Here's the drawing with two shaded views (mm, measured from the low corner). I have some questions. Give positions to 0.01 mm unless a question says otherwise; leave off trailing zeros. Loops run counter-clockwise (first coordinate to the right, second up) from the corner with the lowest first, then second, coordinate; pieces in that order, holes last. Notation, with made-up numbers: M -32.5,79.5 L 11.5,79.5 A25 ccw 11.5,97.5 Z; hole C 37,53 d4. An arc over 180 degrees is marked long. Write item = value, one per line. Start each with the question number.
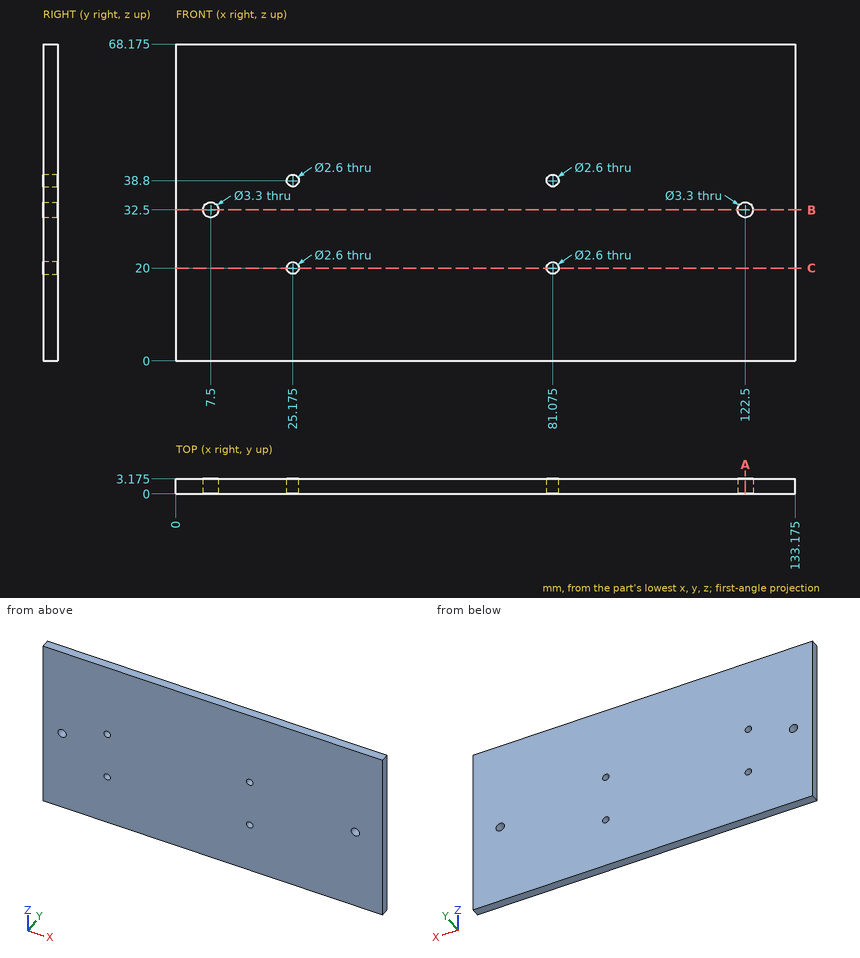
Q1. If we section it at B-B, the plane z = 32.5: List the corners of the cut face in (x, y) for me (3 decimals), then the cut area to 3 significant figures.
Q2. If I drill on line 1 along X through (y, z) = (1.15, 32.5) (3 decimals); line 2 along X through (y, z) = (1.15, 38.8) (3 decimals), over which ranges is the centre line in solid material (lowest first)?
Q3. If we section it at C-C, the plane z = 20: List the corners of the cut face in (x, y) for me (3 decimals).
Q4. Will this pin go through, and if not, where does the flat tip stop? pin 1 (1.6 mm diameter, centred on x = 25.175, z = 38.8, fed in from -Y).
Q5. If we section it at A-A, the plane x = 122.5: List the corners of the cut face in (y, z) for me (3 decimals).
Resolved:
q1.outline = M 0,0 L 5.85,0 L 5.85,3.175 L 0,3.175 Z; M 9.15,0 L 120.85,0 L 120.85,3.175 L 9.15,3.175 Z; M 124.15,0 L 133.175,0 L 133.175,3.175 L 124.15,3.175 Z
q1.area = 402 mm²
q2.line_1 = 0 to 5.85, 9.15 to 120.85, 124.15 to 133.175
q2.line_2 = 0 to 23.875, 26.475 to 79.775, 82.375 to 133.175
q3.outline = M 0,0 L 23.875,0 L 23.875,3.175 L 0,3.175 Z; M 26.475,0 L 79.775,0 L 79.775,3.175 L 26.475,3.175 Z; M 82.375,0 L 133.175,0 L 133.175,3.175 L 82.375,3.175 Z
q4.pin_1 = through
q5.outline = M 0,0 L 3.175,0 L 3.175,30.85 L 0,30.85 Z; M 0,34.15 L 3.175,34.15 L 3.175,68.175 L 0,68.175 Z
